Verification items for the finished model (mm, model axes). A direction names the side the tool comes from. Give positions to 0.01 mm unless a question says otherwise; leave off trailing zeros. Order: outer loops, then holes, each group sorted by start corner. A loop starts at its lowest first (then second) coordinate and runs counter-clockwise, first axis right, second up. Notation, with made-up numbers: (47.5, 1) -> (77.5, 1) arc R7 ccw to (77.5, 10) -> close; hole circle Ø5 at (-0.5, 89). An arc over 180 degrees is marked (long way). Return JSON: item names as keys, results as strings. Group by question number.
(1) Tool access check on faces 4 (the face through (0, 11.112, 50)), 5 (the face through (0, 12.7, 50)). Record the directions out of +Z, -Z, +X, -X, +Y, -Y that give a thin tool (end or side, any length) a straight path to the whole face; none if there is none.
(2) Depth check by flat-ended pin: pin 1 Ø5.5 at (y, z) = (4.76, 95.25) entering from +X. Enter the tip coordinate at first touch or a pass-through.
(3) Cross-section at A-A on x = 2.75. Enter the section's corners in (y, z).
(4) Release check for a two-part mould opening along Y. For faces 1 (the face through (0, -12.7, 50)), 2 (the face through (-11.9, 0.14, 34.92)), 3 (the face through (-11.3, 0.1, 101.6)) record: pulls with the +Y half, pulls with the -Y half, needs draft (parallel to the pull), parting line crosses it, or undercut.
(5) Cross-section at C-C on y = 0. Enter the section's corners in (x, z) (1 decimal), then the cut area to 3 significant figures.
(6) Cross-section at B-B on z = 31.75. Enter the section's corners in (x, y) (1 decimal).
(7) Cross-section at D-D on z = 95.25. Enter the section's corners in (x, y).
(8) Thickness scan on line 1 along Y through (x, z) = (-12, 95.25); line 2 along Y through (x, z) = (12.4, 31.75) (3 decimals); line 3 along X through (y, z) = (-3.25, 78). Record the ranges inside material, lowest first.
from build123d import *

# Parameters (mm, degrees)
SKETCH1_W           = 25.4
SKETCH1_H           = 25.4
SKETCH1_W_2         = 22.225
SKETCH1_H_2         = 22.225
BOSS_EXTRUDE1_DEPTH = 101.6
SKETCH2_R           = 2.38125
SKETCH2_R_2         = 3.175
CUT_EXTRUDE1_DEPTH  = 25.4


with BuildPart() as part:
    # Sketch1 → Boss-Extrude1 (new body)
    with BuildSketch(Plane.XY):
        Rectangle(SKETCH1_W, SKETCH1_H)
        Rectangle(SKETCH1_W_2, SKETCH1_H_2, mode=Mode.SUBTRACT)
    extrude(amount=BOSS_EXTRUDE1_DEPTH)

    # Sketch2 → Cut-Extrude1 (cut)
    with BuildSketch(Plane(origin=(12.7, 0, 0), x_dir=(0, 0, -1), z_dir=(1, 0, 0))):
        with Locations((-95.25, 4.7625)):
            Circle(SKETCH2_R)
        with Locations((-95.25, -4.7625)):
            Circle(SKETCH2_R)
        with Locations((-31.75, 0)):
            Circle(SKETCH2_R_2)
    extrude(amount=-CUT_EXTRUDE1_DEPTH, mode=Mode.SUBTRACT)


solid = part.part
Verdict:
{
 "1": {"face 4": "+Z, -Z", "face 5": "+Z, -Z, +X, -X, +Y"},
 "2": {"pin 1": "x = 12.7"},
 "3": {"outline": "(-12.7, 0) -> (-11.11, 0) -> (-11.11, 101.6) -> (-12.7, 101.6) -> close; (11.11, 0) -> (12.7, 0) -> (12.7, 101.6) -> (11.11, 101.6) -> close"},
 "4": {"face 1": "pulls with the -Y half", "face 2": "undercut", "face 3": "needs draft"},
 "5": {"outline": "(-12.7, 0) -> (-11.1, 0) -> (-11.1, 28.6) -> (-12.7, 28.6) -> close; (-12.7, 34.9) -> (-11.1, 34.9) -> (-11.1, 101.6) -> (-12.7, 101.6) -> close; (11.1, 0) -> (12.7, 0) -> (12.7, 28.6) -> (11.1, 28.6) -> close; (11.1, 34.9) -> (12.7, 34.9) -> (12.7, 101.6) -> (11.1, 101.6) -> close", "area": "302 mm²"},
 "6": {"outline": "(-12.7, -12.7) -> (12.7, -12.7) -> (12.7, -3.2) -> (11.1, -3.2) -> (11.1, -11.1) -> (-11.1, -11.1) -> (-11.1, -3.2) -> (-12.7, -3.2) -> close; (-12.7, 3.2) -> (-11.1, 3.2) -> (-11.1, 11.1) -> (11.1, 11.1) -> (11.1, 3.2) -> (12.7, 3.2) -> (12.7, 12.7) -> (-12.7, 12.7) -> close"},
 "7": {"outline": "(-12.7, -12.7) -> (12.7, -12.7) -> (12.7, -7.14) -> (11.11, -7.14) -> (11.11, -11.11) -> (-11.11, -11.11) -> (-11.11, -7.14) -> (-12.7, -7.14) -> close; (-12.7, -2.38) -> (-11.11, -2.38) -> (-11.11, 2.38) -> (-12.7, 2.38) -> close; (-12.7, 7.14) -> (-11.11, 7.14) -> (-11.11, 11.11) -> (11.11, 11.11) -> (11.11, 7.14) -> (12.7, 7.14) -> (12.7, 12.7) -> (-12.7, 12.7) -> close; (11.11, -2.38) -> (12.7, -2.38) -> (12.7, 2.38) -> (11.11, 2.38) -> close"},
 "8": {"line 1": "-12.7 to -7.14, -2.38 to 2.38, 7.14 to 12.7", "line 2": "-12.7 to -3.175, 3.175 to 12.7", "line 3": "-12.7 to -11.11, 11.11 to 12.7"}
}
